CAD build for the part. Positions are in the model's coordinates, mm. Face numbers are marked on the shaded views. A direction names the side the tool comes from. Coordinates: 2 decimals unless noted, no trailing zeros. Loops run counter-clockwise (first coordinate to the right, second up) from the corner with the lowest first, then second, coordinate; pieces in that order, holes last. Notation, with made-up numbers: (25, -25.5) -> (58, -25.5) arc R20 ccw to (58, -18.5) -> close; hole circle Ø4 at (-3.75, 75.25). An arc over 180 degrees is marked (long way). Answer as CSV lines item,"result". Start each with the question number.
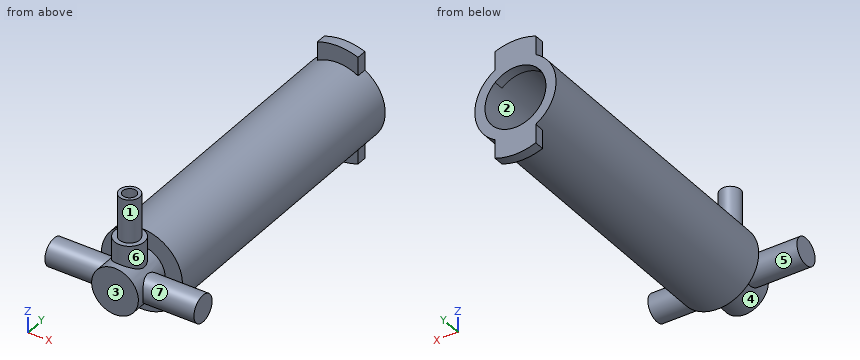
from build123d import *

# Parameters (mm, degrees)
SKETCH1_R           = 6
BOSS_EXTRUDE1_DEPTH = 44.5
SHELL1_T            = -1.5
SKETCH3_R           = 3.45
BOSS_EXTRUDE3_DEPTH = 5.9
SHELL2_START        = -4.4
SHELL2_OUTLINE_R    = 1.95
SHELL2_DEPTH        = 5.9
SKETCH5_R           = 2.2
BOSS_EXTRUDE4_DEPTH = 6.4
SKETCH6_R           = 1.5
BOSS_EXTRUDE5_DEPTH = 6.4
SKETCH7_R           = 1
CUT_EXTRUDE1_DEPTH  = 12.4
SKETCH8_R           = 1.95
CUT_EXTRUDE2_DEPTH  = 51.902357509
SKETCH9_R           = 2
BOSS_EXTRUDE6_DEPTH = 11
SKETCH10_R          = 1.975
CUT_EXTRUDE3_DEPTH  = 52.730551947
SKETCH11_R          = 1
CUT_EXTRUDE4_DEPTH  = 12
BOSS_EXTRUDE9_DEPTH = 1.5


# Read off the part's stored shape, not the designer's step: Shell2
with BuildPart() as part:
    # Sketch1 → Boss-Extrude1 (new body)
    with BuildSketch(Plane(origin=(0, 0, 0), x_dir=(1, 0, 0), z_dir=(0, 1, 0))):
        with Locations(Location((0, 0, 0), (0, 0, 270))):
            Circle(SKETCH1_R)
    extrude(amount=BOSS_EXTRUDE1_DEPTH)

    # Shell1
    shell1_openings = [part.faces().sort_by_distance(p)[0] for p in [
        (0, 44.5, 0),
    ]]
    offset(amount=SHELL1_T, openings=shell1_openings, kind=Kind.INTERSECTION)

    # Sketch3 → Boss-Extrude3 (add)
    with BuildSketch(Plane.XZ):
        with Locations(Location((0, 0, 0), (0, 0, 270))):
            Circle(SKETCH3_R)
    extrude(amount=BOSS_EXTRUDE3_DEPTH)

    # Shell2 outline → Shell2 (cut)
    with BuildSketch(Plane(origin=(0, 0, 0), x_dir=(1, 0, 0), z_dir=(0, 1, 0)).offset(SHELL2_START)):
        Circle(SHELL2_OUTLINE_R)
    extrude(amount=SHELL2_DEPTH, mode=Mode.SUBTRACT)

    # Sketch5 → Boss-Extrude4 (add)
    with BuildSketch(Plane.XY):
        with Locations(Location((0, -2.70320485, 0), (0, 0, 270))):
            Circle(SKETCH5_R)
    extrude(amount=BOSS_EXTRUDE4_DEPTH)

    # Sketch6 → Boss-Extrude5 (add)
    with BuildSketch(Plane.XY.offset(6.4)):
        with Locations((0, -2.70320485)):
            Circle(SKETCH6_R)
    extrude(amount=BOSS_EXTRUDE5_DEPTH)

    # Sketch7 → Cut-Extrude1 (cut)
    with BuildSketch(Plane.XY.offset(12.8)):
        with Locations((0, -2.70320485)):
            Circle(SKETCH7_R)
    extrude(amount=-CUT_EXTRUDE1_DEPTH, mode=Mode.SUBTRACT)

    # Sketch8 → Cut-Extrude2 (cut, through all)
    with BuildSketch(Plane(origin=(0, -4.4, 0), x_dir=(1, 0, 0), z_dir=(0, 1, 0))):
        with Locations(Location((0, 0, 0), (0, 0, 270))):
            Circle(SKETCH8_R)
    extrude(amount=CUT_EXTRUDE2_DEPTH, mode=Mode.SUBTRACT)

    # Sketch9 → Boss-Extrude6 (add)
    with BuildSketch(Plane(origin=(0, 0, 0), x_dir=(0, 0, -1), z_dir=(1, 0, 0))):
        with Locations(Location((0, -2.934503104, 0), (0, 0, 180))):
            Circle(SKETCH9_R)
    extrude(amount=BOSS_EXTRUDE6_DEPTH)

    # Sketch10 → Cut-Extrude3 (cut, through all)
    with BuildSketch(Plane(origin=(0, -4.4, 0), x_dir=(1, 0, 0), z_dir=(0, 1, 0))):
        with Locations(Location((0, -0.025, 0), (0, 0, 270))):
            Circle(SKETCH10_R)
    extrude(amount=CUT_EXTRUDE3_DEPTH, mode=Mode.SUBTRACT)

    # Sketch11 → Cut-Extrude4 (cut)
    with BuildSketch(Plane.XY.offset(12.8)):
        with Locations((0, -2.70320485)):
            Circle(SKETCH11_R)
    extrude(amount=-CUT_EXTRUDE4_DEPTH, mode=Mode.SUBTRACT)

    # Mirror5: part across plane


with BuildPart() as part_1:
    add(part.part)
    add(part.part.mirror(Plane(origin=(0, 0, 0), x_dir=(0, 0, 1), z_dir=(1, 0, 0))))

    # Sketch14 → Boss-Extrude9 (add)
    with BuildSketch(Plane(origin=(0, 44.5, 0), x_dir=(1, 0, 0), z_dir=(0, 1, 0))):
        with BuildLine():
            Line((-3, -3.346313625), (-3, -7.95298686))
            ThreePointArc((-3, -7.95298686), (0, -8.5), (3, -7.95298686))
            Line((3, -7.95298686), (3, -3.346313625))
            ThreePointArc((3, -3.346313625), (0, -4.494197912), (-3, -3.346313625))
        make_face()
        with BuildLine():
            Line((3, 3.346313625), (3, 7.95298686))
            ThreePointArc((3, 7.95298686), (0, 8.5), (-3, 7.95298686))
            Line((-3, 7.95298686), (-3, 3.346313625))
            ThreePointArc((-3, 3.346313625), (0, 4.494197912), (3, 3.346313625))
        make_face()
    extrude(amount=-BOSS_EXTRUDE9_DEPTH)


solid = part_1.part
Item 1: Wall check: probe 1 along X at (y, z) = (30.5, 0); probe 2 along Z at (x, y) = (0, -0.7); probe 3 along Y at (x, z) = (0, 9.75). Give the ranges that are in metal, low to high.
Item 2: Flat gauge pins, fed straight in: pin 1 Ø4 at (y, z) = (31, 1.5) entering from -X; pin 2 Ø2.5 at (x, z) = (0, -7.5) entering from -Y; pin 3 Ø5 at (x, y) = (0, 17.5) entering from -Z; pin 4 Ø4 at (x, z) = (5.5, 7.5) entering from +Y. Where does each tip first touch, or does it go through?
Item 3: Saw through at C-C (z = 9). Write the cut outline in (x, y), plus the area to 3 significant figures.
Item 4: Two-plate mould, pull along Y, no slides. Class the marked faces 1, 2, 3 and 4: pulls with the +Y half, pulls with the -Y half, needs draft (parallel to the pull), parting line crosses it, or undercut.
Item 5: Which spindle directions (+Z, -Z, +X, -X, +Y, -Y) get a long thin tool onto all of the face, cutting with end or side? Do the marked faces 5, 6 and 7. Say none if no direction does.
Item 6: Saw through at A-A (y = 12). Write the cut outline in (x, z), plus the area to 3 significant figures.
Item 7: Saw through at B-B (z = 0). Write the cut outline in (x, y).
Geometry check:
1,probe 1,"-6 to -4.5, 4.5 to 6"
1,probe 2,"-3.45 to -1.95, 2 to 6.4"
1,probe 3,"-4.2 to -3.7, -1.7 to -1.2"
2,pin 1,"x = -6"
2,pin 2,"y = 43"
2,pin 3,"z = -6"
2,pin 4,"through"
3,outline,"circle Ø3 at (0, -2.7); hole circle Ø2 at (0, -2.7)"
3,area,"3.93 mm2"
4,face 1,"undercut"
4,face 2,"needs draft"
4,face 3,"pulls with the -Y half"
4,face 4,"undercut"
5,face 5,"-X"
5,face 6,"+Z"
5,face 7,"+X"
6,outline,"circle Ø12 at (0, 0); hole circle Ø9 at (0, 0)"
6,area,"49.5 mm2"
7,outline,"(-11, -4.93) -> (-3.45, -4.93) -> (-3.45, -5.9) -> (3.45, -5.9) -> (3.45, -4.93) -> (11, -4.93) -> (11, -0.93) -> (3.45, -0.93) -> (3.45, 0) -> (6, 0) -> (6, 44.5) -> (4.5, 44.5) -> (4.5, 1.5) -> (1.97, 1.5) -> (1.97, -4.4) -> (-1.97, -4.4) -> (-1.97, 1.5) -> (-4.5, 1.5) -> (-4.5, 44.5) -> (-6, 44.5) -> (-6, 0) -> (-3.45, 0) -> (-3.45, -0.93) -> (-11, -0.93) -> close"
